Check sheet for the modelled part. Datum: model origin and axes. Units: mm. A direction names the side the tool comes from. Give positions to 0.01 mm unless a question says otherwise; leave off trailing zeros. Write each loop counter-clockwise with the first axis right and the second up, starting at its lowest first coordinate (ties: lowest second). Pieces come first, ordered by that corner, then holes. Notation, with made-up numbers: M 63.25,17.5 L 95.25,17.5 A19 cw 95.25,21.5 Z; hole C 19,-2 d9. An arc over 180 degrees is marked long. Write item = value, one per line. Start each with the question number.
1) Mould release check, pull along X, two halves, no side actions. Record for faces 3 (the cylindrical face through (97.26, 0.52, -51.26)), 4 (the cylindrical face through (96.9, 0.5, -50.9)), 5 (the cylindrical face through (-13.1, 0.5, -51.6)), 6 (the cylindrical face through (96.615, 0.501, -8.265)): released by +X, released by -X, zero draft, split by the parting line, or undercut.
2) Cross-section at B-B, the plane x = 43.5. Record the cut outline in (y, z), plus the area to 3 significant figures.
3) Cross-section at A-A, the plane z = -24. Record the cut outline in (x, y).
4) Cross-section at C-C, the plane y = 0.7. Record the cut outline in (x, z).
5) Access from +Z, -Z, +X, -X, +Y, -Y to the whole of each face (thin tool, end or side, straight path). Record for faces 1 (the cylindrical face through (96.97, 0.52, -7.9)), 2 (the cylindrical face through (-12.79, 0.5, -51.19)).
6) Scan lines: line 1 along Z through (x, y) = (8, 0.7); line 2 along X through (y, z) = (0.35, -26); line 3 along X through (y, z) = (0.7, -44.5). Record each from-to range of solid material in increasing order. Write a range as [from, to].
```python
from build123d import *

# Parameters (mm, degrees)
BOSS_EXTRUDE1_DEPTH = 1.016
CUT_EXTRUDE7_DEPTH  = 2.54


with BuildPart() as part:
    # Sketch1 → Boss-Extrude1 (new body)
    with BuildSketch(Plane(origin=(0, 0, 0), x_dir=(1, 0, 0), z_dir=(0, 1, 0))):
        with BuildLine():
            Line((0, 0), (83.82, 0))
            ThreePointArc((83.82, 0), (98.912902724, 6.251685004), (105.164587728, 21.344587728))
            Line((105.164587728, 21.344587728), (105.164587728, 38.108587728))
            ThreePointArc((105.164587728, 38.108587728), (98.912902724, 53.201490452), (83.82, 59.453175456))
            Line((83.82, 59.453175456), (0, 59.453175456))
            ThreePointArc((0, 59.453175456), (-15.092902724, 53.201490452), (-21.344587728, 38.108587728))
            Line((-21.344587728, 38.108587728), (-21.344587728, 21.344587728))
            ThreePointArc((-21.344587728, 21.344587728), (-15.092902724, 6.251685004), (0, 0))
        make_face()
        with BuildLine():
            Line((0, 3.048), (83.82, 3.048))
            ThreePointArc((83.82, 3.048), (96.757641255, 8.406946473), (102.116587728, 21.344587728))
            Line((102.116587728, 21.344587728), (102.116587728, 38.108587728))
            ThreePointArc((102.116587728, 38.108587728), (96.757641255, 51.046228983), (83.82, 56.405175456))
            Line((83.82, 56.405175456), (0, 56.405175456))
            ThreePointArc((0, 56.405175456), (-12.937641255, 51.046228983), (-18.296587728, 38.108587728))
            Line((-18.296587728, 38.108587728), (-18.296587728, 21.344587728))
            ThreePointArc((-18.296587728, 21.344587728), (-12.937641255, 8.406946473), (0, 3.048))
        make_face(mode=Mode.SUBTRACT)
    extrude(amount=BOSS_EXTRUDE1_DEPTH)

    # Sketch6 → Cut-Extrude7 (cut)
    with BuildSketch(Plane(origin=(0, 1.016, 0), x_dir=(1, 0, 0), z_dir=(0, 1, 0))):
        with BuildLine():
            Line((0, 0), (83.82, 0))
            ThreePointArc((83.82, 0), (98.912902724, 6.251685004), (105.164587728, 21.344587728))
            Line((105.164587728, 21.344587728), (105.164587728, 38.108587728))
            ThreePointArc((105.164587728, 38.108587728), (98.912902724, 53.201490452), (83.82, 59.453175456))
            Line((83.82, 59.453175456), (0, 59.453175456))
            ThreePointArc((0, 59.453175456), (-15.092902724, 53.201490452), (-21.344587728, 38.108587728))
            Line((-21.344587728, 38.108587728), (-21.344587728, 21.344587728))
            ThreePointArc((-21.344587728, 21.344587728), (-15.092902724, 6.251685004), (0, 0))
        make_face()
        with BuildLine():
            Line((0, 2.54), (83.82, 2.54))
            ThreePointArc((83.82, 2.54), (97.1168515, 8.047736228), (102.624587728, 21.344587728))
            Line((102.624587728, 21.344587728), (102.624587728, 38.108587728))
            ThreePointArc((102.624587728, 38.108587728), (97.1168515, 51.405439228), (83.82, 56.913175456))
            Line((83.82, 56.913175456), (0, 56.913175456))
            ThreePointArc((0, 56.913175456), (-13.2968515, 51.405439228), (-18.804587728, 38.108587728))
            Line((-18.804587728, 38.108587728), (-18.804587728, 21.344587728))
            ThreePointArc((-18.804587728, 21.344587728), (-13.2968515, 8.047736228), (0, 2.54))
        make_face(mode=Mode.SUBTRACT)
    extrude(amount=-CUT_EXTRUDE7_DEPTH, mode=Mode.SUBTRACT)


solid = part.part
```
Reply:
q1.face_3 = released by +X
q1.face_4 = undercut
q1.face_5 = released by -X
q1.face_6 = undercut
q2.outline = M 0,-56.91 L 1.02,-56.91 L 1.02,-56.41 L 0,-56.41 Z; M 0,-3.05 L 1.02,-3.05 L 1.02,-2.54 L 0,-2.54 Z
q2.area = 1.03 mm2
q3.outline = M -18.8,0 L -18.3,0 L -18.3,1.02 L -18.8,1.02 Z; M 102.12,0 L 102.62,0 L 102.62,1.02 L 102.12,1.02 Z
q4.outline = M -18.8,-38.11 A18.8 ccw 0,-56.91 L 83.82,-56.91 A18.8 ccw 102.62,-38.11 L 102.62,-21.34 A18.8 ccw 83.82,-2.54 L 0,-2.54 A18.8 ccw -18.8,-21.34 Z; hole M -18.3,-38.11 A18.3 ccw 0,-56.41 L 83.82,-56.41 A18.3 ccw 102.12,-38.11 L 102.12,-21.34 A18.3 ccw 83.82,-3.05 L 0,-3.05 A18.3 ccw -18.3,-21.34 Z
q5.face_1 = +Z, +X, +Y, -Y
q5.face_2 = +Y, -Y
q6.line_1 = [-56.91, -56.41], [-3.05, -2.54]
q6.line_2 = [-18.8, -18.3], [102.12, 102.62]
q6.line_3 = [-17.69, -17.14], [100.96, 101.51]
